Geometry: final body of the model. Coordinates: model frame, mm. Face numbers are marked on the shaded views. A direction names the side the tool comes from. Round coordinates to 2 decimals unless told otherwise and drop trailing zeros. Order: outer loops, then holes, each group sorted by start corner. A loop starts at its lowest first (then second) coordinate and runs counter-clockwise, first axis right, second up. Notation, with made-up numbers: M -12.5,64 L 32.5,64 A31 cw 32.5,95 Z; hole C -28.75,33.25 d1. An arc over 180 degrees is marked long. Return JSON: item names as keys, results as strings. Group by question number.
Q1. Mould query, pull axis X, two halves, no side actions, for the marked faces 6, 7 and 8. Classes: released by +X, released by -X, zero draft, split by the parting line, or undercut.
Q2. Cut plane B-B on y = 13. Output: boundary loops of the cut face in (x, z), and give its area (3 significant figures).
Q3. Access query for the marked faces 1, 2, 3, 4 and 5. Directions: +Z, -Z, +X, -X, +Y, -Y. A direction counts if a zero-diameter tool reaches every point of the face in a straight line with its end or side. Return the directions, or none.
Q4. Contact query for flat-ended pins moving along their axis: pin 1 (8 mm diameter, centred on x = 12, y = 13.5, fed in from -Z); pin 2 (6 mm diameter, centred on x = 81, y = 0.5, fed in from +Z); pin 3 (6 mm diameter, centred on y = 1.5, z = -28.5, fed in from -X). Output: stop coordinate, or through.
Q5. Cut plane A-A on y = 0.5. Output: boundary loops of the cut face in (x, z).
Q6. Ray query, probe 1 along Z at (x, y) = (42.5, 2); probe 2 along X at (y, z) = (-10, -45); probe 3 along X at (y, z) = (10, -4). Return the intervals inside material, ascending.
Q7. Cut plane D-D on x = 67.5. Output: boundary loops of the cut face in (y, z), and give its area (3 significant figures).
Q8. Cut plane C-C on z = -11. Output: boundary loops of the cut face in (x, y).
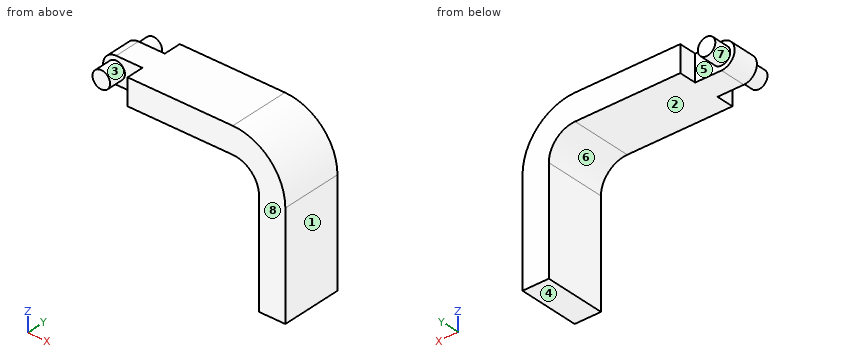
```python
from build123d import *

# Parameters (mm, degrees)
EXTRUDE_1_DEPTH      = 7.5
EXTRUDE_1_DEPTH_BACK = 7.5
SKETCH_1_R           = 5
SKETCH_2_R           = 5
EXTRUDE_2_DEPTH      = 17.5
EXTRUDE_3_DEPTH      = 10


with BuildPart() as part:
    # Sketch 1 → Extrude 1 (new, two sides: drawn at the far end of the back side and taken through both)
    with BuildSketch(Plane(origin=(0, 0, 0), x_dir=(1, 0, 0), z_dir=(0, 1, 0)).offset(-EXTRUDE_1_DEPTH_BACK)):
        with BuildLine():
            Line((0, 0), (75, 0))
            ThreePointArc((75, 0), (96.213203436, 8.786796564), (105, 30))
            Line((105, 30), (105, 90))
            Line((105, 90), (90.00000671, 90))
            Line((90.00000671, 90), (90.00000671, 30))
            ThreePointArc((90.00000671, 30), (85.606608428, 19.393398282), (75.00000671, 15))
            Line((75.00000671, 15), (0, 15))
            ThreePointArc((0, 15), (-7.5, 7.5), (0, 0))
        make_face()
        with Locations(Location((0, 7.5, 0), (0, 0, 270))):
            Circle(SKETCH_1_R, mode=Mode.SUBTRACT)
    extrude(amount=EXTRUDE_1_DEPTH + EXTRUDE_1_DEPTH_BACK)

    # Sketch 2 → Extrude 2 (add, symmetric)
    with BuildSketch(Plane(origin=(0, 0, 0), x_dir=(1, 0, 0), z_dir=(0, 1, 0))):
        with Locations(Location((0, 7.5, 0), (0, 0, 270))):
            Circle(SKETCH_2_R)
    extrude(amount=EXTRUDE_2_DEPTH, both=True)

    # Sketch 3 → Extrude 3 (add)
    with BuildSketch(Plane(origin=(0, 7.5, 0), x_dir=(1, 0, 0), z_dir=(0, 1, 0))):
        with BuildLine():
            Line((90.00000671, 90), (90.00000671, 30))
            ThreePointArc((90.00000671, 30), (85.606608428, 19.393398282), (75.00000671, 15))
            Line((75.00000671, 15), (15.00000671, 15))
            Line((15.00000671, 15), (15.00000671, 0))
            Line((15.00000671, 0), (75, 0))
            ThreePointArc((75, 0), (96.213203436, 8.786796564), (105, 30))
            Line((105, 30), (105, 90))
            Line((105, 90), (90.00000671, 90))
        make_face()
    extrude_3 = extrude(amount=EXTRUDE_3_DEPTH)

    # Mirror 1: Extrude 3 across plane
    add(extrude_3.mirror(Plane.ZX))


solid = part.part
```
Result sheet:
{
 "1": {"face 6": "released by -X", "face 7": "undercut", "face 8": "zero draft"},
 "2": {"outline": "C 0,-7.5 d10; M 15,-15 L 75,-15 A15 cw 90,-30 L 90,-90 L 105,-90 L 105,-30 A30 ccw 75,0 L 15,0 Z", "area": "2,410 mm²"},
 "3": {"face 1": "+Z, -Z, +X, +Y, -Y", "face 2": "-Z, -X, +Y, -Y", "face 3": "-Y", "face 4": "-Z, +X, -X, +Y, -Y", "face 5": "+Y"},
 "4": {"pin 1": "stops at z = -15", "pin 2": "stops at z = -0.15", "pin 3": "stops at x = 89.31"},
 "5": {"outline": "M 0,-15 L 75,-15 A15 cw 90,-30 L 90,-90 L 105,-90 L 105,-30 A30 ccw 75,0 L 0,0 A7.5 ccw Z"},
 "6": {"probe 1": "z = -15 to 0", "probe 2": "x = 90 to 105", "probe 3": "x = -3.57 to 3.57, 15 to 89.97"},
 "7": {"outline": "M -17.5,-15 L 17.5,-15 L 17.5,0 L -17.5,0 Z", "area": "525 mm²"},
 "8": {"outline": "M -6.63,-7.5 L -3.57,-7.5 L -3.57,-17.5 L 3.57,-17.5 L 3.57,-7.5 L 15,-7.5 L 15,-17.5 L 98.22,-17.5 L 98.22,17.5 L 15,17.5 L 15,7.5 L 3.57,7.5 L 3.57,17.5 L -3.57,17.5 L -3.57,7.5 L -6.63,7.5 Z"}
}
